Can you work these out from the model? Positions are in its coordinate system, mm. Face numbers are marked on the shaded views. Coordinates: 2 decimals unless noted, no trailing zeros. Order: outer loops, then holes, each group sorted by start corner. A loop starts at its lowest first (then second) coordinate and runs counter-clockwise, first axis right, second up. Notation, with made-up numbers: (81.25, 87) - (103.25, 87) arc R29 cw to (103.25, 116) - close; hole circle Ø8 at (-18.75, 38). An arc over 180 degrees is marked (long way). Return JSON: item names as keys, results as strings. Group by question number.
1) Imagine slicing it at A-A (y = -4). Write out the boundary of the cut face in (x, z).
2) If we mould it in two halves opening along X, with no side actions, what happens to the marked faces 1, 2 and 3? For each: pulls with the +X half, pulls with the -X half, needs draft (parallel to the pull), parting line crosses it, or undercut.
3) If I drill on line 1 along Z through (x, y) = (0, 8.25); line 2 along Y through (x, z) = (4, 6.5) (3 decimals); line 3 along X through (y, z) = (7.75, 6.35), over which ranges is the centre line in solid material (lowest first)?
4) Imagine slicing it at D-D (x = 5). Write out the boundary of the cut face in (y, z) (3 decimals).
5) Imagine slicing it at B-B (x = -3.5). Write out the boundary of the cut face in (y, z) (3 decimals).
6) Imagine slicing it at C-C (y = -1.5). Write out the boundary of the cut face in (x, z), and give its area (3 significant figures).
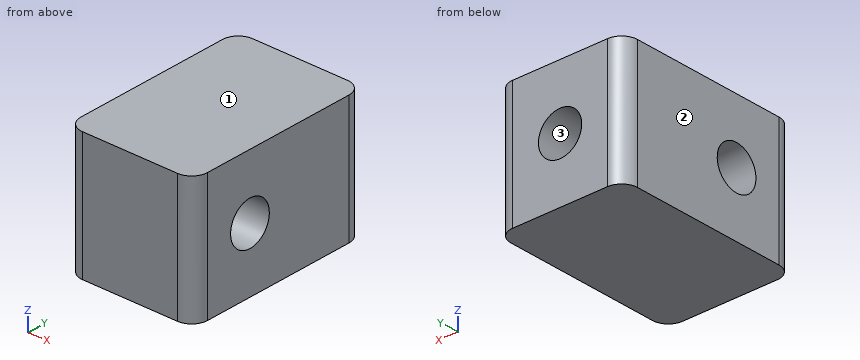
Autodesk Inventor part; units mm, degrees
ref_plane "YZ Plane" through (0, 0, 0) normal (1, 0, 0) x (0, 1, 0)
ref_plane "XZ Plane" through (0, 0, 0) normal (0, 1, 0) x (-1, 0, 0)
ref_plane "XY Plane" through (0, 0, 0) normal (0, 0, 1) x (1, 0, 0)
sketch "Sketch1" plane through (0, 0, 0) normal (0, 0, 1) x (1, 0, 0)
  line L0 (6.35, -9.525) -> (-6.35, -9.525)
  line L1 (-6.35, -9.525) -> (-6.35, 9.525)
  line L2 (-6.35, 9.525) -> (6.35, 9.525)
  line L3 (6.35, 9.525) -> (6.35, -9.525)
  line L4 (6.35, -9.525) -> (-6.35, 9.525) construction
  line L5 (-6.35, -9.525) -> (6.35, 9.525) construction
  point P0 (0, 0)
  dimension "d0" = 12.7
  dimension "d1" = 19.05
extrude "Plate1" add sketch "Sketch1" along normal blind 12.7
sketch "Sketch2" plane through (-6.35, 9.525, 0) normal (0, 1, 0) x (1, 0, 0)
  line L0 (12.7, 0) -> (0, 0)
  point P0 (6.35, 0)
  point P1 (6.35, -6.35)
  point P2 (6.35, 0)
  dimension "d3" = 6.35
hole "Hole1" at (0, 9.525, 6.35) direction (0, -1, 0) diameter 4.3434 depth 6.35 tip angle 118
sketch "Sketch3" plane through (6.35, -9.525, 0) normal (1, 0, 0) x (0, 0, -1)
  line L0 (0, 19.05) -> (-12.7, 19.05)
  point P0 (0, 9.525)
  point P1 (-6.35, 6.35)
  point P2 (-6.35, 19.05)
  dimension "d11" = 12.7
hole "Hole2" at (6.35, -3.175, 6.35) direction (-1, 0, 0) diameter 4.3434 depth 12.7
fillet "Corner Round1" radius 1.5875 4 edges at (6.35, 9.525, 6.35) (-6.35, 9.525, 6.35) (-6.35, -9.525, 6.35) (6.35, -9.525, 6.35)
equation "\"d17\" = Thickness"
equation "\"d2\" = Thickness"
equation "\"BendRadius\" = Thickness"
equation "\"BendReliefWidth\" = Thickness"
equation "\"BendReliefDepth\" = 0.5 * Thickness"
equation "\"CornerReliefSize\" = 4 * Thickness"
equation "\"MinimumRemnant\" = 2 * Thickness"
equation "\"TransitionRadius\" = BendRadius"
equation "\"JacobiRadiusSize\" = BendRadius"
equation "\"GapSize\" = Thickness"
properties part number "PLATE,NUT-BLOCK,SINGLE-L" material "Aluminum 6061"
Calculated:
{
 "1": {"outline": "(-6.35, 0) - (6.35, 0) - (6.35, 4.34) - (-6.35, 4.34) - close; (-6.35, 8.36) - (6.35, 8.36) - (6.35, 12.7) - (-6.35, 12.7) - close"},
 "2": {"face 1": "needs draft", "face 2": "pulls with the -X half", "face 3": "undercut"},
 "3": {"line 1": "0 to 4.18, 8.52 to 12.7", "line 2": "-9.525 to -5.342, -1.008 to 9.525", "line 3": "-6.35 to -2.17, 2.17 to 6.35"},
 "4": {"outline": "(-9.507, 0) - (9.507, 0) - (9.507, 12.7) - (-9.507, 12.7) - close; hole circle Ø4.343 at (-3.175, 6.35)"},
 "5": {"outline": "(-9.525, 0) - (9.525, 0) - (9.525, 12.7) - (-9.525, 12.7) - close; hole circle Ø4.343 at (-3.175, 6.35)"},
 "6": {"outline": "(-6.35, 0) - (6.35, 0) - (6.35, 4.97) - (-6.35, 4.97) - close; (-6.35, 7.73) - (6.35, 7.73) - (6.35, 12.7) - (-6.35, 12.7) - close", "area": "126 mm2"}
}
